Answer from the drawing. Dimensions are ordinates in mm from the lowest x, y and z of the part. A direction names the side the tool comes from. Round coordinates to 2 decimals unless told otherwise and drop trailing zeros. Loops run counter-clockwise (first coordinate to the right, second up) from the corner with the lowest first, then second, coordinate; pieces in that order, holes last. Notation, with made-up numbers: M -35.75,-19 L -19.75,-19 A15 cw -19.75,-12 Z; hole C 12,3.25 d11. An arc over 180 degrees is marked long. Write each question's results on one line, items separated by ' | '.
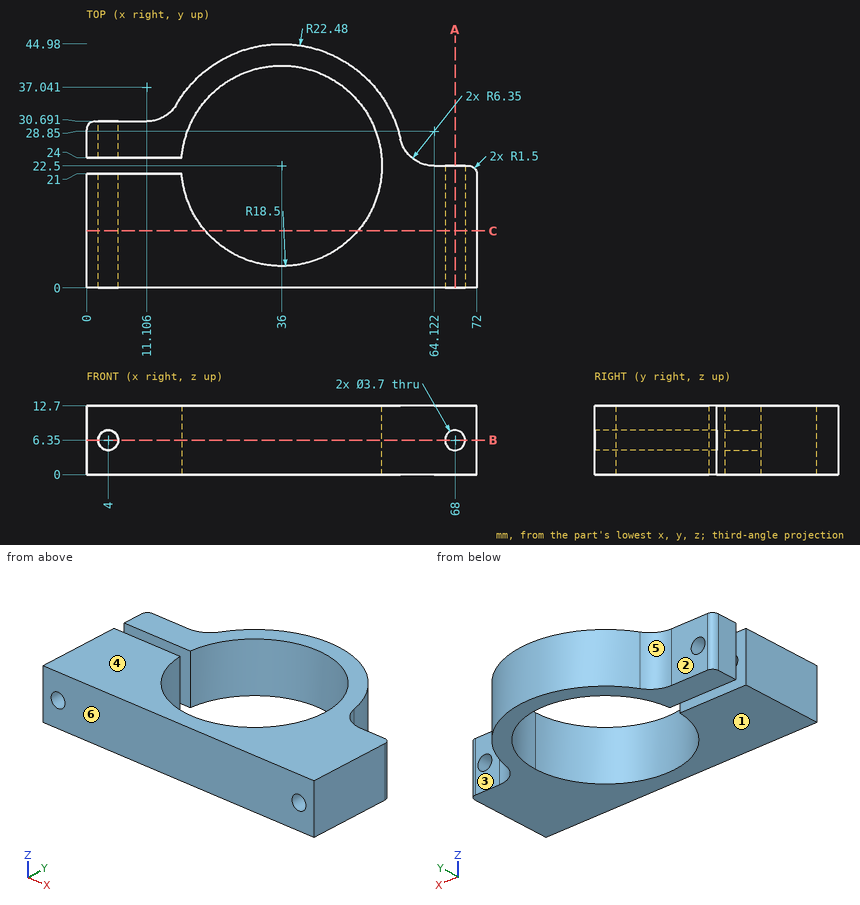
1. Find section B-B, the plane z = 6.35. Count the separate pieces of the cut face and the enclosed holes in it, then the cut area to 3 significant figures.
Completed:
separate pieces: 4 | enclosed holes: 0 | area: 1,220 mm2
2. Find the intervals of material crossed by L1, parallel to Z at x = 4, y = 16; L2, parallel to Y at x = 36, z = 9.5; L3, parallel to X at y = 28, z = 6.35, in increasing order.
Completed:
L1: z = 0 to 4.5, 8.2 to 12.7 | L2: y = 0 to 4, 41 to 44.98 | L3: x = 0 to 2.15, 5.85 to 18.34, 53.66 to 57.8
3. Find section A-A, the plane x = 68. Give the vertices of the cut face in (y, z).
Completed:
outline: M 0,0 L 22.5,0 L 22.5,4.5 L 0,4.5 Z; M 0,8.2 L 22.5,8.2 L 22.5,12.7 L 0,12.7 Z
4. Find section C-C, the plane y = 10.5. Give the vertices of the cut face in (x, z), then the cut area to 3 significant figures.
Completed:
outline: M 0,0 L 21.92,0 L 21.92,12.7 L 0,12.7 Z; M 50.08,0 L 72,0 L 72,12.7 L 50.08,12.7 Z; hole C 4,6.35 d3.7; hole C 68,6.35 d3.7 | area: 535 mm2
5. Which of the six approach directions +Z, -Z, +X, -X, +Y, -Y give full straight-line access (tool end or side, diameter ignored) to the marked faces 1, 2 and 3?
Completed:
face 1: -Z, +X, -X, +Y, -Y | face 2: +Z, -Z, -X, +Y | face 3: +Z, -Z, +X, +Y
6. Given P1, Ø2, axis at x = 4, z = 6.35, coming from the -Y side; P2, Ø3, axis at x = 68.5, z = 6.5, coming from the +Y side; P3, Ø6.5, axis at x = 12.5, z = 6.5, coming from the +Y side; P4, Ø5, axis at x = 4, z = 6.5, coming from the +Y side, each flat-ended and moving along its own axis, determine where each tip first touches the part or whether it passes through.
Completed:
P1: passes through | P2: stops at y = 22.5 | P3: stops at y = 32.71 | P4: stops at y = 30.69
7. Determine the mould class of the marked faces 4, 5 and 6 for opening direction Y: released by +Y, released by -Y, zero draft, split by the parting line, or undercut.
Completed:
face 4: zero draft | face 5: released by +Y | face 6: released by -Y
